Could you check a few things on this model? Use its own coordinates, in mm. A direction names the side the tool comes from. Round coordinates to 2 decimals unless told otherwise and drop trailing zeros. Write each loop counter-clockwise with the first axis right and the second up, starting at its lowest first coordinate (ties: lowest second). Pieces come first, ordered by that corner, then holes. Notation, with made-up numbers: (-25, 49.25) -> (-20, 49.25) arc R30 cw to (-20, 78.25) -> close; hole circle Ø6 at (27.5, 78.25). An arc over 180 degrees is marked (long way). Return JSON: item names as keys, results as strings.
from build123d import *
from build123d import SkipClean  # not in build123d's __all__

# Parameters (mm, degrees)
F1_DEPTH  = 3
F2_R      = 10
F3_R      = 1.5
F4_DEPTH  = 2
F5_DEPTH  = 6
F6_R      = 1.9
F6_R_2    = 1.5
F7_DEPTH  = 1
F9_W      = 1
F9_H      = 10.6840910192
F9_W_2    = 7.2588436306
F9_H_2    = 0.5
F9_W_3    = 6.9682821631
F10_DEPTH = 6


# Not quite as in the source:
# - a fillet or chamfer that OpenCascade refuses, or shapes differently, is made with other operations: its cross-section is extruded or revolved along the edge and cut away or added
# - after a boolean that leaves OpenCascade's solid faulty, fix() repairs it


with BuildPart() as f1:
    # F0 (on Top) → F1 (new body)
    with BuildSketch(Plane.XY):
        Polygon((-45, 2), (-45, 0), (-32.1715728753, 0), (-33, 2), align=None)
        Polygon((-33, 2), (-32.1715728753, 0), (-19.1715728753, 13), (-20, 15), align=None)
        Polygon((-20, 15), (-19.1715728753, 13), (0, 13), (0, 15), align=None)
        Polygon((0, 15), (0, 13), (19.1715728753, 13), (20, 15), align=None)
        Polygon((20, 15), (19.1715728753, 13), (32.1715728753, 0), (33, 2), align=None)
        Polygon((33, 2), (32.1715728753, 0), (45, 0), (45, 2), align=None)
    extrude(amount=F1_DEPTH)

    # F2
    f2_edges = [f1.edges().sort_by_distance(p)[0] for p in [
        (-33, 2, 1.5),
        (-20, 15, 1.5),
        (20, 15, 1.5),
        (33, 2, 1.5),
        (32.171573, 0, 1.5),
        (19.171573, 13, 1.5),
        (-19.171573, 13, 1.5),
        (-32.171573, 0, 1.5),
    ]]
    fillet(f2_edges, radius=F2_R)

    # F3 (on face) → F4 (join, through all)
    with BuildSketch(Plane.XZ):
        with BuildLine():
            Line((-45, 0), (-45, 3))
            ThreePointArc((-45, 3), (-46.5, 1.5), (-45, 0))
        make_face()
        with Locations((45, 1.5)):
            Circle(F3_R)
    extrude(amount=-F4_DEPTH)

    # F3 (on face) → F5 (join)
    with BuildSketch(Plane.XZ):
        with BuildLine():
            Line((-45, 0), (-45, 3))
            ThreePointArc((-45, 3), (-46.5, 1.5), (-45, 0))
        make_face()
        with BuildLine():
            ThreePointArc((-45, 0), (-43.9393398282, 0.4393398282), (-43.5, 1.5))
            ThreePointArc((-43.5, 1.5), (-43.9393398282, 2.5606601718), (-45, 3))
            Line((-45, 3), (-45, 0))
        make_face()
        with Locations((45, 1.5)):
            Circle(F3_R)
    with SkipClean():  # cleaning this boolean's faces spoils the solid; the shape is the same uncleaned
        extrude(amount=F5_DEPTH)

    # F6 (on face) → F7 (join)
    with BuildSketch(Plane.XZ.offset(6)):
        with Locations((-45, 1.5)):
            Circle(F6_R)
        with Locations((-45, 1.5)):
            Circle(F6_R_2, mode=Mode.SUBTRACT)
        with Locations((45, 1.5)):
            Circle(F6_R)
    extrude(amount=-F7_DEPTH)

    add(f1.part.fix(), mode=Mode.REPLACE)

    # F8: fillet of radius 0.5 on 4 edges, made by hand

    # F8_s1 → F8_t2 (revolve, cut)
    with BuildSketch(Plane.XY.offset(1.5)):
        with BuildLine():
            ThreePointArc((-43.1, -5.5), (-43.2464466094, -5.8535533906), (-43.6, -6))
            Line((-43.6, -6), (-43.1, -6))
            Line((-43.1, -6), (-43.1, -5.5))
        make_face()
    revolve(axis=Axis((-45, -6, 1.5), (0, -1, 0)), mode=Mode.SUBTRACT)

    # F8_s3 → F8_t4 (revolve, cut)
    with BuildSketch(Plane.XY.offset(1.5)):
        with BuildLine():
            ThreePointArc((-43.5, -5), (-43.2127016654, -5.1736701825), (-43.1, -5.4898979486))
            Line((-43.1, -5.4898979486), (-43.1, -5))
            Line((-43.1, -5), (-43.5, -5))
        make_face()
    revolve(axis=Axis((-45, -5, 1.5), (0, -1, 0)), mode=Mode.SUBTRACT)

    # F8_s5 → F8_t6 (revolve, cut)
    with BuildSketch(Plane.XY.offset(1.5)):
        with BuildLine():
            ThreePointArc((46.5, -5), (46.7872983346, -5.1736701825), (46.9, -5.4898979486))
            Line((46.9, -5.4898979486), (46.9, -5))
            Line((46.9, -5), (46.5, -5))
        make_face()
    revolve(axis=Axis((45, -5, 1.5), (0, -1, 0)), mode=Mode.SUBTRACT)

    # F8_s7 → F8_t8 (revolve, cut)
    with BuildSketch(Plane.XY.offset(1.5)):
        with BuildLine():
            ThreePointArc((46.9, -5.5), (46.7535533906, -5.8535533906), (46.4, -6))
            Line((46.4, -6), (46.9, -6))
            Line((46.9, -6), (46.9, -5.5))
        make_face()
    revolve(axis=Axis((45, -6, 1.5), (0, -1, 0)), mode=Mode.SUBTRACT)

    # F9 (on face) → F10 (cut, through all)
    with BuildSketch(Plane.XZ.offset(6)):
        with Locations((-45, 1.5)):
            Rectangle(F9_W, F9_H)
        with Locations((-54.3349329382, 3.15)):
            Rectangle(F9_W_2, F9_H_2)
        with Locations((-54.1896522045, -0.15)):
            Rectangle(F9_W_3, F9_H_2)
        with Locations((54.1896522045, -0.15)):
            Rectangle(F9_W_3, F9_H_2)
        with Locations((54.3349329382, 3.15)):
            Rectangle(F9_W_2, F9_H_2)
        with Locations((45, 1.5)):
            Rectangle(F9_W, F9_H)
    extrude(amount=-F10_DEPTH, mode=Mode.SUBTRACT)


solid = f1.part
1) Thinking about a two-plate mould opening in X: for faces 5 (the face through (33.37, 2.74, 1.52)), 6 (the face through (-44.5, -3, 1)), 7 (the face through (0, 14, 0)), which applies, pulls with the +X half, pulls with the -X half, needs draft (parallel to the pull), parting line crosses it, or undercut?
Return value:
{"face 5": "pulls with the +X half", "face 6": "undercut", "face 7": "needs draft"}
2) For faces 1 (the face through (32.44, 0.78, 1.52)), 2 (the face through (46.5, -1.5, 1.5)), 3 (the face through (-46.5, -1.5, 1.5)), 4 (the face through (42, 2, 1)), which set-ups out of +Z, -Z, +X, -X, +Y, -Y let a thin tool reach every point of the face, with its end or its side?
Return value:
{"face 1": "+Z, -Z, -Y", "face 2": "+X, +Y", "face 3": "-X, +Y", "face 4": "+Z, -Z, +X, +Y"}
3) I want a section at C-C, the plane x = 32. Please give me the cut outline in (y, z).
Return value:
{"outline": "(0.98, 0) -> (3.42, 0) -> (3.42, 3) -> (0.98, 3) -> close"}
4) If I drill on probe 1 along X at (y, z) = (-4, 1.45); probe 2 along X at (y, z) = (-2, 2.6); probe 3 along Y at (x, z) = (-2, 0.65), over which ranges is the centre line in solid material (lowest first)? Write a range as [from, to].
Return value:
{"probe 1": "[-46.5, -45.5], [-44.5, -43.5], [43.5, 44.5], [45.5, 46.5]", "probe 2": "[-46.02, -45.5], [-44.5, -43.98], [43.98, 44.5], [45.5, 46.02]", "probe 3": "[13, 15]"}
5) I want a section at B-B, the plane x = 8. Please give me the cut outline in (y, z).
Return value:
{"outline": "(13, 0) -> (15, 0) -> (15, 3) -> (13, 3) -> close"}
6) I want a section at A-A, the plane y = 6. Please give me the cut outline in (x, z), and give its area (3 significant figures).
Return value:
{"outline": "(-29, 0) -> (-26.17, 0) -> (-26.17, 3) -> (-29, 3) -> close; (26.17, 0) -> (29, 0) -> (29, 3) -> (26.17, 3) -> close", "area": "17.0 mm²"}
7) Will these pins go through, and if not, where does the flat tip stop? pin 1 Ø1.1 at (y, z) = (-2, 1) entering from +X; pin 2 Ø2 at (x, z) = (29, 0) entering from +Y; pin 3 Ø2 at (x, z) = (2.5, 2) entering from -Y.
Return value:
{"pin 1": "x = 46.5", "pin 2": "y = 7", "pin 3": "y = 13"}
